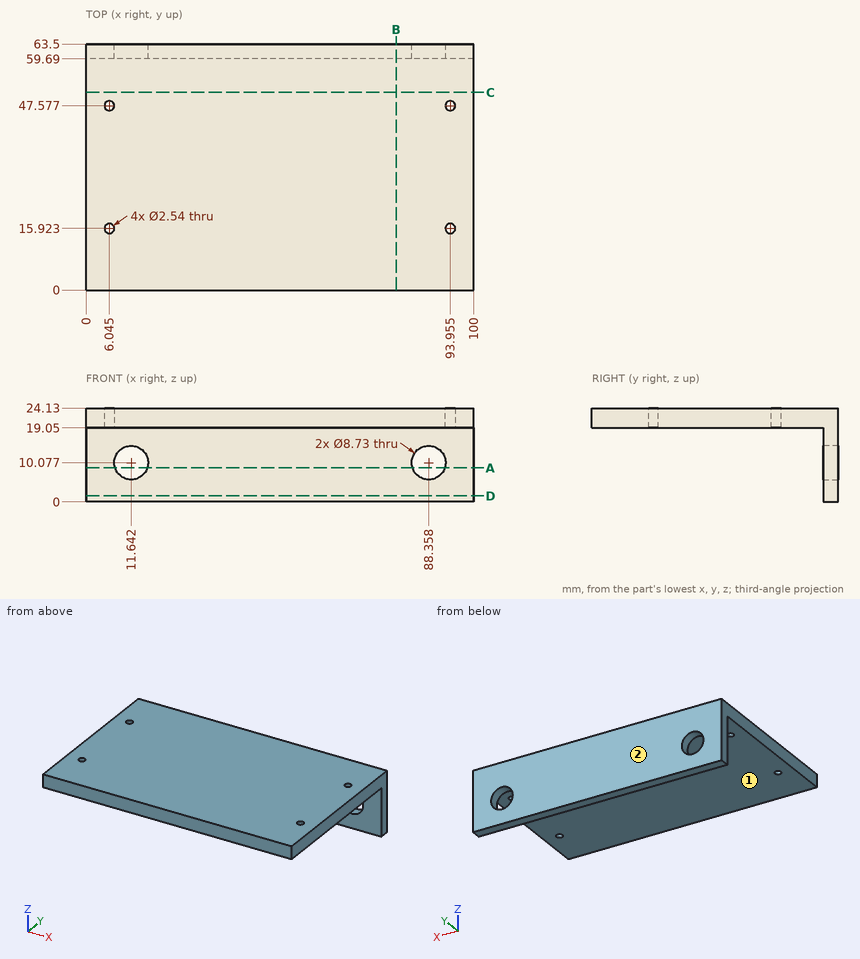
Verification items for this drawing (mm, ordinates from the low corner). A direction names the side the tool comes from. Round coordinates to 2 decimals unless told otherwise and drop trailing zeros. Write each loop counter-clockwise with the first axis right and the second up, starting at its lowest first coordinate (ties: lowest second). Pieces come first, ordered by that corner, then holes. Notation, with made-up numbers: (-24, 19.5) - (-7, 19.5) arc R21 cw to (-7, 47.5) - close; hole circle Ø4 at (62.25, -39.5). An arc over 180 degrees is marked (long way). Answer as a JSON object with one key per item and string values. Group by question number.
Q1. Section check A-A, the plane z = 8.75. Enter the section's corners in (x, y).
Q2. Section check D-D, the plane z = 1.5. Enter the section's corners in (x, y).
Q3. Thickness scan on line 1 (Y direction, x = 5, z = 19.5) (1 decimal); line 2 (Z direction, x = 77.5, y = 8); line 3 (Y direction, x = 71.5, z = 16.25). Record the ranges inside material, lowest first.
Q4. Section check B-B, the plane x = 80. Enter the section's corners in (y, z).
Q5. Tool access check on the marked faces 1 and 2. Record the directions out of +Z, -Z, +X, -X, +Y, -Y that give a thin tool (end or side, any length) a straight path to the whole face; none if there is none.
Q6. Section check C-C, the plane y = 51. Enter the section's corners in (x, z), plus the area to 3 significant figures.
Q7. Go/stop test with flat-tipped pins: pin 1 Ø1.5 at (x, y) = (11, 47) entering from -Z; pin 2 Ø5.5 at (x, z) = (36.5, 10.5) entering from -Y. Record where each tip stops, or that it passes through.
Found:
{
 "1": {"outline": "(0, 59.69) - (7.48, 59.69) - (7.48, 63.5) - (0, 63.5) - close; (15.8, 59.69) - (84.2, 59.69) - (84.2, 63.5) - (15.8, 63.5) - close; (92.52, 59.69) - (100, 59.69) - (100, 63.5) - (92.52, 63.5) - close"},
 "2": {"outline": "(0, 59.69) - (100, 59.69) - (100, 63.5) - (0, 63.5) - close"},
 "3": {"line 1": "y = 0 to 15.2, 16.6 to 46.9, 48.3 to 63.5", "line 2": "z = 19.05 to 24.13", "line 3": "y = 59.69 to 63.5"},
 "4": {"outline": "(0, 19.05) - (59.69, 19.05) - (59.69, 0) - (63.5, 0) - (63.5, 24.13) - (0, 24.13) - close"},
 "5": {"face 1": "-Z, +X, -X, -Y", "face 2": "+Z, -Z, +X, -X, +Y"},
 "6": {"outline": "(0, 19.05) - (100, 19.05) - (100, 24.13) - (0, 24.13) - close", "area": "508 mm^2"},
 "7": {"pin 1": "stops at z = 19.05", "pin 2": "stops at y = 59.69"}
}
